from build123d import *

# Parameters (mm, degrees)
SKETCH_2_R          = 2.6
CUT_EXTRUDE_1_DEPTH = 3


with BuildPart() as part:
    # 草图1 → 旋转1 (revolve)
    with BuildSketch(Plane(origin=(0, 0, 0), x_dir=(0, 0, -1), z_dir=(1, 0, 0))):
        Polygon((0, 10.4), (2.3, 10.4), (2.3, 4.4), (5.5, 4.4), (5.5, 0), (0, 0), align=None)
    revolve(axis=Axis((0, 0, 0), (0, 0, -1)))

    # 草图2 → 切除-拉伸1 (cut)
    with BuildSketch(Plane(origin=(0, 0, -5.5), x_dir=(-1, 0, 0), z_dir=(0, 0, -1))):
        Circle(SKETCH_2_R)
    extrude(amount=-CUT_EXTRUDE_1_DEPTH, mode=Mode.SUBTRACT)


solid = part.part
Model file for the job. Use its own axes, mm. A direction names the side the tool comes from. Give positions to 0.01 mm unless a question says otherwise; leave off trailing zeros. Order: outer loops, then holes, each group sorted by start corner. A loop starts at its lowest first (then second) coordinate and runs counter-clockwise, first axis right, second up. Notation, with made-up numbers: (63.5, -36.75) - (91.5, -36.75) arc R15 ccw to (91.5, -22.75) - close; hole circle Ø4 at (55.25, -29). An arc over 180 degrees is marked (long way). Return JSON: item names as keys, results as strings.
1) Cut at D-D, the plane y = 3. Give the cut face in (x, z), plus the area to 3 significant figures.
Geometry says:
{"outline": "(-9.96, -2.3) - (-3.22, -2.3) - (-3.22, -5.5) - (3.22, -5.5) - (3.22, -2.3) - (9.96, -2.3) - (9.96, 0) - (-9.96, 0) - close", "area": "66.4 mm²"}
2) Cut at A-A, the plane x = 0. Give the cut face in (y, z).
Geometry says:
{"outline": "(-10.4, -2.3) - (-4.4, -2.3) - (-4.4, -5.5) - (-2.6, -5.5) - (-2.6, -2.5) - (2.6, -2.5) - (2.6, -5.5) - (4.4, -5.5) - (4.4, -2.3) - (10.4, -2.3) - (10.4, 0) - (-10.4, 0) - close"}
3) Probe line 1 (Z direction, x = 2.25, y = 6.25); line 2 (X direction, y = -0.5, z = -5.2); line 3 (Y direction, x = 3.75, z = -1.7). List the from-to ranges inside material, lowest first. Write a range as from..to.
Geometry says:
{"line 1": "-2.3..0", "line 2": "-4.37..-2.55, 2.55..4.37", "line 3": "-9.7..9.7"}
4) Cut at C-C, the plane z = -3.95. Give the cut face in (x, y).
Geometry says:
{"outline": "circle Ø8.8 at (0, 0); hole circle Ø5.2 at (0, 0)"}
5) 3-axis set-ups, long thin cutter, end or side, ignore diameter. For faces 1 (the flat face through (0, 0, -2.5)), 2 (the cylindrical face through (10.31, -1.35, -1.17)): which of +Z, -Z, +X, -X, +Y, -Y reach the whole face in a straight line?
Geometry says:
{"face 1": "-Z", "face 2": "+Z, -Z"}
6) Flat gauge pins, fed straight in: P1, Ø1.5, axis at y = -1, z = -4, coming from the -X side; P2, Ø1.5, axis at x = -1, z = -2.5, coming from the +Y side; P3, Ø2.5, axis at x = -1, y = 0, coming from the -Z side. Where does each tip first touch, or does it go through?
Geometry says:
{"P1": "x = -4.39", "P2": "y = 10.4", "P3": "z = -2.5"}
